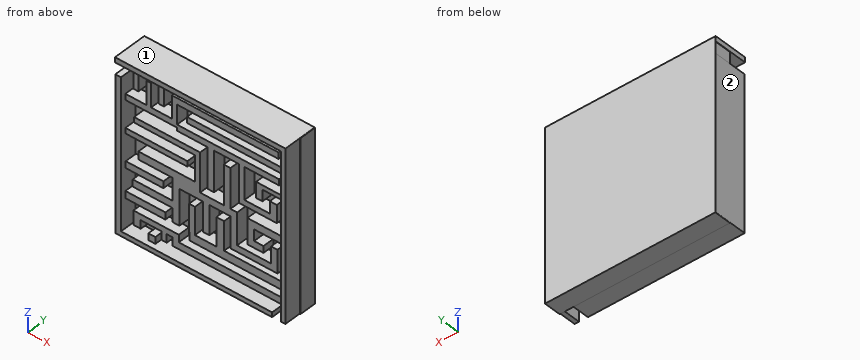
from build123d import *

# Parameters (mm, degrees)
F0_W     = 100
F0_H     = 100
F3_DEPTH = 10
F1_W     = 2.5462172925
F1_H     = 96.7562794685
F1_W_2   = 88.7259021401
F1_H_2   = 2.7420781553
F4_DEPTH = 20
F2_W     = 2.9379464686
F2_H     = 12.5352256
F2_W_2   = 2.5462172925
F2_H_2   = 13.9062739909
F2_W_3   = 3.9172582328
F2_H_3   = 23.699412588
F2_W_4   = 59.5423225313
F2_H_4   = 3.7213973701
F2_W_5   = 4.1131153703
F2_H_5   = 7.0510646328
F2_W_6   = 3.1338073313
F2_H_6   = 13.3186765015
F2_W_7   = 57.7795598656
F2_H_7   = 3.5255327821
F2_W_8   = 3.7213899195
F2_H_8   = 6.6593382508
F2_W_9   = 5.4841600358
F2_H_9   = 3.9172582328
F2_H_10  = 23.2097543776
F2_H_11  = 9.7931455821
F2_W_10  = 3.7213945761
F2_H_12  = 17.2359370627
F2_W_11  = 35.7449837029
F2_H_13  = 3.1338054687
F2_W_12  = 23.3076885343
F2_H_14  = 4.1131218895
F2_W_13  = 4.504846409
F2_H_15  = 16.8442111462
F2_W_14  = 62.480266206
F2_W_15  = 2.9379427433
F2_H_16  = 4.8965737224
F2_W_16  = 4.3089836836
F2_W_17  = 36.4305013791
F2_H_17  = 3.1338064
F2_W_18  = 22.1325084567
F2_W_19  = 23.503549397
F2_H_18  = 4.1131190956
F2_W_20  = 4.1131209582
F5_DEPTH = 17


with BuildPart() as f3:
    # F0 (on Front) → F3 (new body)
    with BuildSketch(Plane.XZ):
        with Locations((5.8758892119, 4.0513307203)):
            Rectangle(F0_W, F0_H)
    extrude(amount=F3_DEPTH)

    # F1 (on face) → F4 (join)
    with BuildSketch(Plane.XZ):
        Polygon((55.7230003178, 54.1560947895), (-44.3629510701, 54.1560947895), (-44.3629510701, 51.2181520462), (53.1767830253, 51.2181520462), (55.7230003178, 51.2181520462), align=None)
        with Locations((54.4498916715, 2.8400123119)):
            Rectangle(F1_W, F1_H)
        Polygon((-44.167086482, 44.5588119328), (-44.167086482, -45.7339882851), (-40.837418288, -45.7339882851), (-40.837418288, -42.9919101298), (-40.837418288, 44.5588119328), align=None)
        with Locations((3.5255327821, -44.3629492074)):
            Rectangle(F1_W_2, F1_H_2)
    extrude(amount=F4_DEPTH)

    # F2 (on face) → F5 (join)
    with BuildSketch(Plane.XZ):
        with Locations((-34.6677359194, 44.9505392462)):
            Rectangle(F2_W, F2_H)
        Polygon((-40.837418288, 33.3946235478), (-40.837418288, 29.869094491), (-10.4786660522, 29.869094491), (-10.4786660522, 31.6318590194), (-10.4786660522, 33.3946235478), (-13.4166097268, 33.3946235478), (-25.7559735328, 33.3946235478), (-28.3021908253, 33.3946235478), align=None)
        Polygon((-10.4786660522, 31.6318590194), (-10.4786660522, 29.869094491), (-10.4786660522, 28.1063281), (7.3448577896, 28.1063281), (11.2621160224, 28.1063281), (25.7559753954, 28.1063281), (29.0856454521, 28.1063281), (49.4553856552, 28.1063281), (49.4553856552, 31.6318590194), align=None)
        with Locations((-27.0290821791, 40.3477605432)):
            Rectangle(F2_W_2, F2_H_2)
        Polygon((-13.4166097268, 33.3946235478), (-10.4786660522, 33.3946235478), (-10.4786660522, 42.9919101298), (-10.4786660522, 46.7133074999), (-13.4166097268, 46.7133074999), align=None)
        with Locations((9.303486906, 16.256621806)):
            Rectangle(F2_W_3, F2_H_3)
        with Locations((19.2924952134, 44.8526088148)):
            Rectangle(F2_W_4, F2_H_4)
        Polygon((29.0856454521, 9.3034887686), (29.0856454521, 28.1063281), (25.7559753954, 28.1063281), (25.7559753954, 5.9738187119), (29.0856454521, 5.9738187119), align=None)
        Polygon((43.9712256193, 9.3034887686), (29.0856454521, 9.3034887686), (29.0856454521, 5.9738187119), (48.0843409896, 5.9738187119), (48.0843409896, 9.3034887686), align=None)
        with Locations((46.0277833045, 12.8290210851)):
            Rectangle(F2_W_5, F2_H_5)
        with Locations((-19.6842234582, 44.5588137954)):
            Rectangle(F2_W_6, F2_H_6)
        with Locations((24.2870030925, 37.3118855059)):
            Rectangle(F2_W_7, F2_H_7)
        Polygon((53.372643888, 20.6635370851), (53.372643888, 23.2097543776), (35.9408482909, 23.2097543776), (35.9408482909, 20.6635370851), (39.6622382104, 20.6635370851), align=None)
        with Locations((37.8015432507, 17.3338679597)):
            Rectangle(F2_W_8, F2_H_8)
        Polygon((53.372643888, -4.4069155119), (53.372643888, 0), (30.8484081179, 0), (30.8484081179, -4.4069155119), (34.7656644881, -4.4069155119), align=None)
        Polygon((34.7656644881, -4.4069155119), (30.8484081179, -4.4069155119), (30.8484081179, -14.9835133925), (34.7656644881, -14.9835133925), (34.7656644881, -11.0662551597), align=None)
        with Locations((37.507744506, -13.0248842761)):
            Rectangle(F2_W_9, F2_H_9)
        Polygon((24.7766599059, -18.7049079686), (24.7766599059, 0), (20.8594016731, 0), (20.8594016731, -4.2110527866), (20.8594016731, -22.4263034761), (24.7766599059, -22.4263034761), align=None)
        Polygon((20.8594016731, -4.2110527866), (20.8594016731, 0), (16.9421434402, 0), (3.0358759686, 0), (0, 0), (0, -4.2110527866), (4.7986414284, -4.2110527866), (8.5200360045, -4.2110527866), align=None)
        with Locations((18.9007725567, 11.6048771888)):
            Rectangle(F2_W_3, F2_H_10)
        Polygon((44.7546802461, -18.7049079686), (24.7766599059, -18.7049079686), (24.7766599059, -22.4263034761), (48.4760701656, -22.4263034761), (48.4760701656, -18.7049079686), align=None)
        with Locations((46.6153752059, -13.8083351776)):
            Rectangle(F2_W_8, F2_H_11)
        with Locations((6.6593387164, -12.8290213179)):
            Rectangle(F2_W_10, F2_H_12)
        Polygon((0, 0), (3.0358759686, 0), (3.0358759686, 22.8180289268), (0, 22.8180289268), (0, 19.6842234582), (0, 4.6027782373), align=None)
        Polygon((-13.2207460701, 0), (0, 0), (0, 4.6027782373), (-33.1987626851, 4.6027782373), (-33.1987626851, 0), align=None)
        Polygon((0, -4.2110527866), (0, 0), (-13.2207460701, 0), (-13.2207460701, -4.2110527866), (-9.1076260433, -4.2110527866), align=None)
        with Locations((-17.8724918514, 21.2511261925)):
            Rectangle(F2_W_11, F2_H_13)
        Polygon((-9.1076260433, -25.168383494), (-9.1076260433, -4.2110527866), (-13.2207460701, -4.2110527866), (-13.2207460701, -13.0248842761), (-13.2207460701, -17.1380061656), (-13.2207460701, -25.168383494), align=None)
        with Locations((-24.8745903373, -15.0814452209)):
            Rectangle(F2_W_12, F2_H_14)
        Polygon((53.1767830253, -30.4566826671), (53.1767830253, -25.7559735328), (17.138004303, -25.7559735328), (12.633157894, -25.7559735328), (12.633157894, -30.4566826671), align=None)
        with Locations((14.8855810985, -17.3338679597)):
            Rectangle(F2_W_13, F2_H_15)
        Polygon((12.633157894, -30.4566826671), (12.633157894, -25.7559735328), (0, -25.7559735328), (-3.2317389268, -25.7559735328), (-3.2317389268, -30.4566826671), align=None)
        Polygon((-3.2317389268, -25.7559735328), (0, -25.7559735328), (0, -9.6952142194), (-3.4276025835, -9.6952142194), (-3.4276025835, -25.7559735328), align=None)
        Polygon((-9.499351494, -30.4566826671), (-13.0248842761, -30.4566826671), (-13.0248842761, -33.7863527238), (-13.0248842761, -38.6829264462), (-9.499351494, -38.6829264462), (-9.499351494, -34.7656682134), align=None)
        Polygon((-13.0248842761, -33.7863527238), (-13.0248842761, -30.4566826671), (-36.1367091537, -30.4566826671), (-36.1367091537, -33.7863527238), (-31.8277254701, -33.7863527238), (-19.4883588701, -33.7863527238), (-16.5504161268, -33.7863527238), align=None)
        with Locations((21.740781609, -36.7242973298)):
            Rectangle(F2_W_14, F2_H_9)
        with Locations((-18.0193874985, -36.234639585)):
            Rectangle(F2_W_15, F2_H_16)
        with Locations((-33.9822173119, -36.234639585)):
            Rectangle(F2_W_16, F2_H_16)
        with Locations((-22.6221675985, 12.4372956343)):
            Rectangle(F2_W_17, F2_H_17)
        with Locations((-29.5752994716, -6.7572705448)):
            Rectangle(F2_W_18, F2_H_9)
        with Locations((-29.0856435895, -23.8952748477)):
            Rectangle(F2_W_19, F2_H_18)
        with Locations((-25.2663167194, -40.8374201506)):
            Rectangle(F2_W_20, F2_H_9)
    extrude(amount=F5_DEPTH)


solid = f3.part
Input: part model. Units: mm. Frame: model coordinates. Face numbers are marked on the shaded views. A direction names the side the tool comes from. Round coordinates to 2 decimals unless told otherwise and drop trailing zeros. Order: outer loops, then holes, each group sorted by start corner. A loop starts at its lowest first (then second) coordinate and runs counter-clockwise, first axis right, second up. Notation, with made-up numbers: (-39, 31) - (10, 31) arc R8 ccw to (10, 37) - close; hole circle Ø9 at (84.5, -9.75). An arc over 180 degrees is marked (long way). Use a Markdown table: item, result.
1. Material intervals for probe 1 along Z at (x, y) = (-14.5, -18); probe 2 along X at (y, z) = (-17.5, -23); probe 3 along Y at (x, z) = (11, -29), sorted ascending.
Evaluation:
| item | result |
|---|---|
| probe 1 | -45.73 to -42.99, 51.22 to 54.16 |
| probe 2 | -44.17 to -40.84, 53.18 to 55.72 |
| probe 3 | -17 to 0 |
2. Section A-A on z = 26. Return the cut outline in (x, y), then the cut area to 3 significant figures.
Evaluation:
| item | result |
|---|---|
| outline | (-44.17, -20) - (-40.84, -20) - (-40.84, -10) - (7.34, -10) - (7.34, -17) - (11.26, -17) - (11.26, -10) - (25.76, -10) - (25.76, -17) - (29.09, -17) - (29.09, -10) - (53.18, -10) - (53.18, -20) - (55.72, -20) - (55.72, -10) - (55.88, -10) - (55.88, 0) - (-44.17, 0) - close |
| area | 1,110 mm^2 |
3. Access query for the marked faces 1 and 2. Directions: +Z, -Z, +X, -X, +Y, -Y. A direction counts if a zero-diameter tool reaches every point of the face in a straight line with its end or side. Return the directions, or none.
Evaluation:
| item | result |
|---|---|
| face 1 | +Z, +X, -X, +Y, -Y |
| face 2 | -Z, -X, +Y, -Y |
4. First-contact query: pin 1 (1.2 mm diameter, centred on y = -12.5, z = -7, fed in from +X); pin 2 (2 mm diameter, centred on x = 22.5, y = -13, fed in from -Z); pin 3 (8 mm diameter, centred on x = 45, z = 25.5, fed in from +Y); pin 4 (3.5 mm diameter, centred on y = -12, z = -33.5, fed in from -X). Flat tips, straight axial feed; report the tip coordinate or a pass-through.
Evaluation:
| item | result |
|---|---|
| pin 1 | x = 55.72 |
| pin 2 | z = -45.73 |
| pin 3 | y = 0 |
| pin 4 | x = -44.17 |
5. Section C-C on y = -13. State how many separate pieces and enclosed holes the cut face has, then the cut area to 3 significant figures.
Evaluation:
| item | result |
|---|---|
| separate pieces | 6 |
| enclosed holes | 0 |
| area | 4,590 mm^2 |
